Answer from the drawing. Dimensions are ordinates in mm from the lowest x, y and z of the part. A direction names the side the tool comes from. Give positions to 0.01 mm unless a question says otherwise; leave off trailing zeros. Loops run counter-clockwise (first coordinate to the right, second up) from the corner with the lowest first, then second, coordinate; pieces in that order, holes last. Notation, with made-up numbers: M 16.5,-35 L 43.5,-35 A15 cw 43.5,-31 Z; hole C 49.5,-11 d8. An arc over 180 degrees is marked long. Use a Markdown table: item, result.
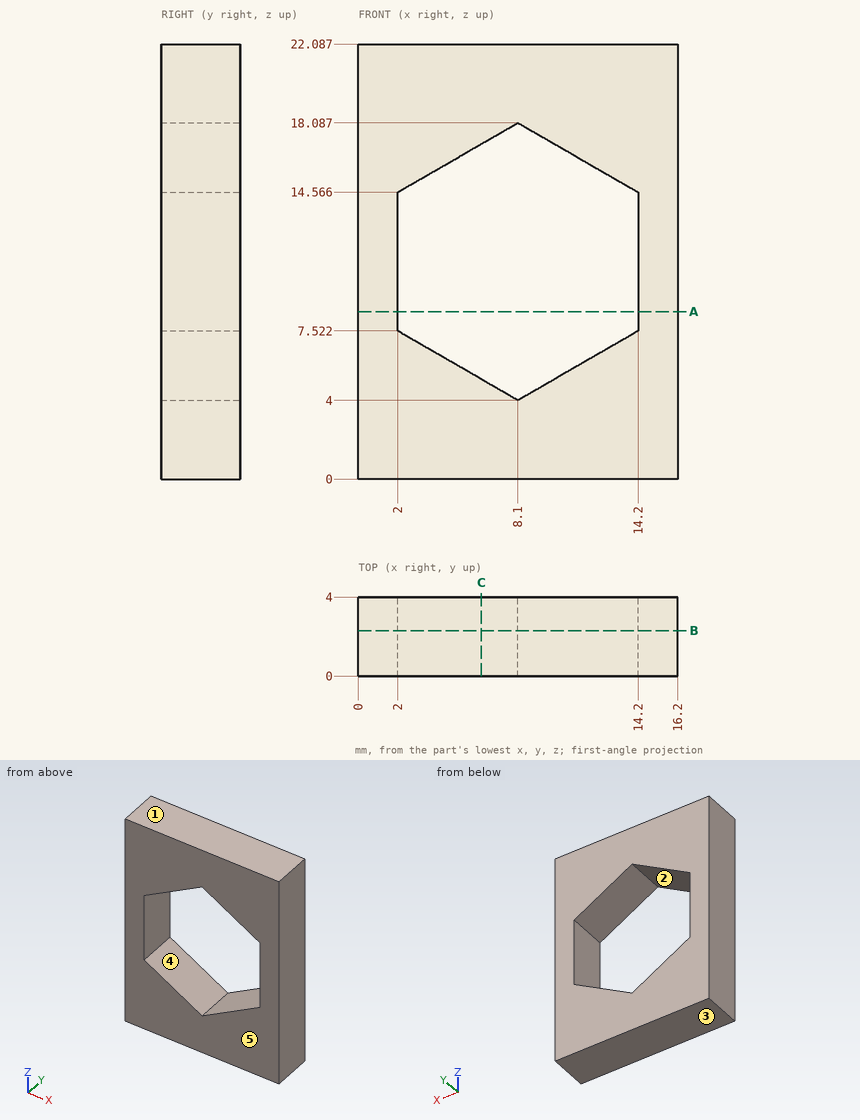
(1) The mould has two halves that part along Z. Classify the marked faces 1, 2 and 3: released by +Z, released by -Z, zero draft, split by the parting line, or undercut.
Entries:
| item | result |
|---|---|
| face 1 | released by +Z |
| face 2 | undercut |
| face 3 | released by -Z |
(2) A cutting plane is placed at C-C (x = 6.25). Write down the section's boundary in (y, z).
Entries:
| item | result |
|---|---|
| outline | M 0,0 L 4,0 L 4,5.07 L 0,5.07 Z; M 0,17.02 L 4,17.02 L 4,22.09 L 0,22.09 Z |
(3) Which of the six approach directions +Z, -Z, +X, -X, +Y, -Y give full straight-line access (tool end or side, diameter ignored) to the marked faces 4 and 5?
Entries:
| item | result |
|---|---|
| face 4 | +Y, -Y |
| face 5 | +Z, -Z, +X, -X, -Y |
(4) Consider probe 1 along X at (y, z) = (0.5, 8.5); probe 2 along Z at (x, y) = (10.5, 0.55) (1 decimal); probe 3 along Z at (x, y) = (8, 2.85). Determine where each line is inside the solid, lowest interval first. Write a range as [from, to].
Entries:
| item | result |
|---|---|
| probe 1 | x = [0, 2], [14.2, 16.2] |
| probe 2 | z = [0, 5.4], [16.7, 22.1] |
| probe 3 | z = [0, 4.06], [18.03, 22.09] |
(5) A cutting plane is placed at B-B (y = 2.3). Write down the section's boundary in (x, z) (1 decimal), and give its area (3 significant figures).
Entries:
| item | result |
|---|---|
| outline | M 0,0 L 16.2,0 L 16.2,22.1 L 0,22.1 Z; hole M 2,7.5 L 8.1,4 L 14.2,7.5 L 14.2,14.6 L 8.1,18.1 L 2,14.6 Z |
| area | 229 mm² |
(6) A cutting plane is placed at A-A (z = 8.5). Write down the section's boundary in (x, y), and give its area (3 significant figures).
Entries:
| item | result |
|---|---|
| outline | M 0,0 L 2,0 L 2,4 L 0,4 Z; M 14.2,0 L 16.2,0 L 16.2,4 L 14.2,4 Z |
| area | 16.0 mm² |
